Geometry: see drawing. Coordinates: mm, zero at the bounding-box minimum. A direction names the side the tool comes from. Give positions to 0.01 mm unless a question says otherwise; leave off trailing zeros. Loops run counter-clockwise (first coordinate to the right, second up) from the corner with the lowest first, then second, coordinate; pieces in that order, holes last. Notation, with made-up numbers: M 15,-19.75 L 44,-19.75 A11 ccw 44,-15.75 Z; hole C 88.25,74 d2. An arc over 180 degrees is marked long. Put each result on its own line as item: value.
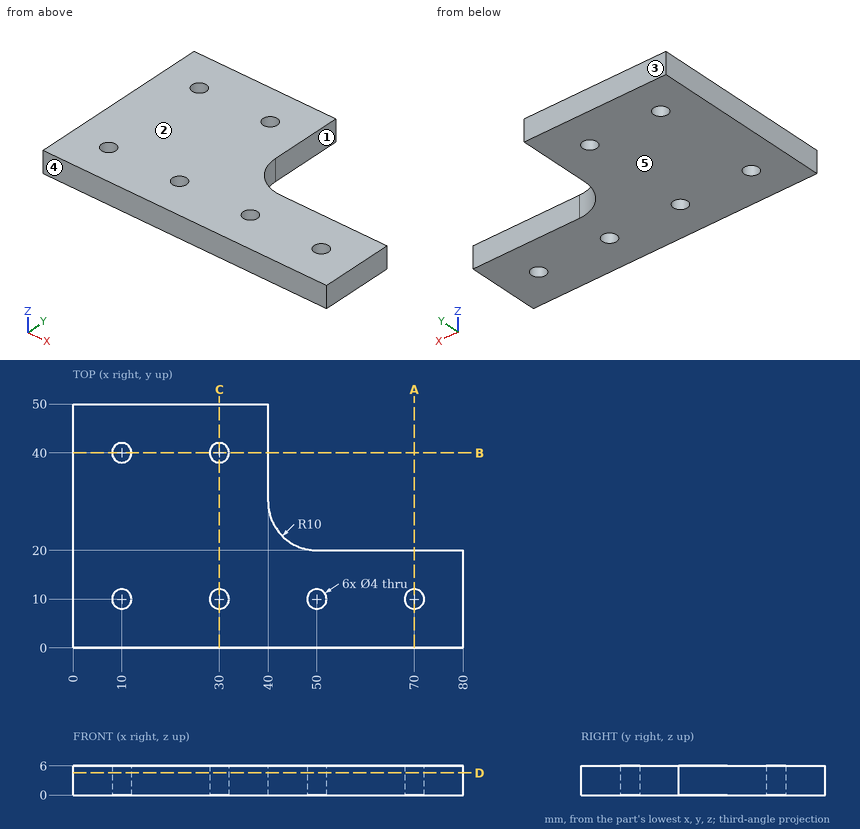
Item 1: Section C-C on x = 30. Output: boundary loops of the cut face in (y, z).
Output values:
outline: M 0,0 L 8,0 L 8,6 L 0,6 Z; M 12,0 L 38,0 L 38,6 L 12,6 Z; M 42,0 L 50,0 L 50,6 L 42,6 Z
Item 2: Line query: probe 1 along Y at (x, z) = (10, 3.65); probe 2 along Y at (x, z) = (70, 1.35); probe 3 along Y at (x, z) = (73, 2.4). Output: solid intervals per line, ascending. Write a range as [from, to].
Output values:
probe 1: [0, 8], [12, 38], [42, 50]
probe 2: [0, 8], [12, 20]
probe 3: [0, 20]
Item 3: Mould query, pull axis Y, two halves, no side actions, for the marked faces 3, 4 and 5. Classes: pulls with the +Y half, pulls with the -Y half, needs draft (parallel to the pull), parting line crosses it, or undercut.
Output values:
face 3: pulls with the +Y half
face 4: pulls with the -Y half
face 5: needs draft
Item 4: Section D-D on z = 4.55. Output: boundary loops of the cut face in (x, y).
Output values:
outline: M 0,0 L 80,0 L 80,20 L 50,20 A10 cw 40,30 L 40,50 L 0,50 Z; hole C 10,10 d4; hole C 10,40 d4; hole C 30,10 d4; hole C 30,40 d4; hole C 50,10 d4; hole C 70,10 d4
Item 5: Section A-A on x = 70. Output: boundary loops of the cut face in (y, z), then the cut area to 3 significant figures.
Output values:
outline: M 0,0 L 8,0 L 8,6 L 0,6 Z; M 12,0 L 20,0 L 20,6 L 12,6 Z
area: 96.0 mm²
Item 6: Pin query (flat end, axial travel): pin 1 Ø6 at (x, y) = (44, 41) entering from -Z (1 decimal); pin 2 Ø3 at (y, z) = (38.5, 4) entering from +X; pin 3 Ø3 at (x, z) = (72.5, 2) entering from +Y. Return the tip coordinate at first contact, or that it passes through.
Output values:
pin 1: through
pin 2: x = 40
pin 3: y = 20
Item 7: Section B-B on y = 40. Output: boundary loops of the cut face in (x, z).
Output values:
outline: M 0,0 L 8,0 L 8,6 L 0,6 Z; M 12,0 L 28,0 L 28,6 L 12,6 Z; M 32,0 L 40,0 L 40,6 L 32,6 Z
Item 8: Set-up query: the marked faces 1 and 2. Return all of +Z, -Z, +X, -X, +Y, -Y with unobstructed straight access to the full face (end or side cutting, diameter ignored); none if empty.
Output values:
face 1: +Z, -Z, +X, +Y
face 2: +Z, +X, -X, +Y, -Y
